from build123d import *

# Parameters (mm, degrees)
F1_DEPTH = 25.4
F2_R     = 7.2533857786
F2_R_2   = 5.5158705089
F2_R_3   = 6.7589997369
F2_R_4   = 6.3667286832
F2_R_5   = 6.9837940253
F2_R_6   = 6.9770855285
F3_DEPTH = 102.87
F4_R     = 5.2099395751
F5_DEPTH = 102.108
F9_START = 96.774
F9_DEPTH = 10.668


with BuildPart() as f1:
    # F0 (on Front) → F1 (new body)
    with BuildSketch(Plane.XZ):
        Polygon((-29.1519459024, 14.0827481248), (-26.7719905823, -18.2049516588), (2.3799553201, -32.2876997836), (29.1519459024, -14.0827481248), (26.7719905823, 18.2049516588), (-2.3799553201, 32.2876997836), align=None)
    extrude(amount=F1_DEPTH)

    # F2 (on Front) → F3 (join)
    with BuildSketch(Plane.XZ):
        with Locations((-28.9137475193, 13.9214349911)):
            Circle(F2_R)
        with Locations((-26.7719905823, -18.2049516588)):
            Circle(F2_R_2)
        with Locations((2.2947418038, -32.2793722153)):
            Circle(F2_R_3)
        with Locations((28.6077819765, -14.5333660766)):
            Circle(F2_R_4)
        with Locations((26.4660213143, 18.5109190643)):
            Circle(F2_R_5)
        with Locations((-2.9066735879, 32.5853340328)):
            Circle(F2_R_6)
    extrude(amount=F3_DEPTH)

    # F4 (on Front) → F5 (join)
    with BuildSketch(Plane.XZ):
        Circle(F4_R)
    extrude(amount=F5_DEPTH)

    # F6 (on Top) → F7 (revolve)
    with BuildSketch(Plane.XY):
        with BuildLine():
            Line((0, -67.7234342558), (0, -29.2267018693))
            ThreePointArc((0, -29.2267018693), (-19.2483661933, -48.4750680625), (0, -67.7234342558))
        make_face()
    revolve(axis=Axis((0, -48.4750680625, 0), (0, -1, 0)))

    # F8 (on Front) → F9 (join)
    with BuildSketch(Plane.XZ.offset(F9_START)):
        Polygon((-28.5810061773, 13.7057788732), (-26.1600557715, -17.8989879787), (2.4209504058, -31.6047668519), (28.5810061773, -13.7057788732), (26.1600557715, 17.8989879787), (-2.4209504058, 31.6047668519), align=None)
    extrude(amount=F9_DEPTH)


solid = f1.part
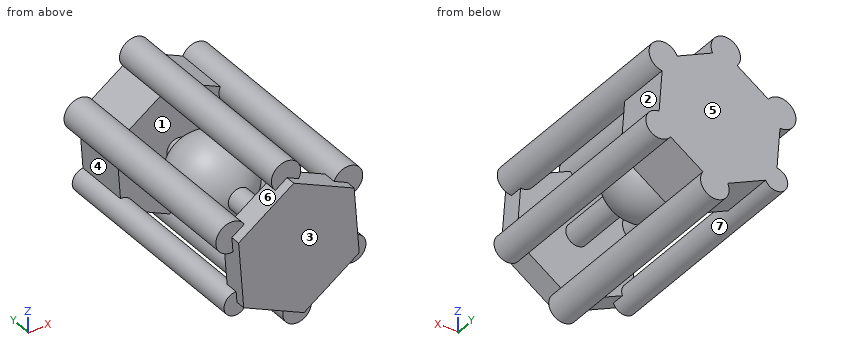
Source: CAD feature listing. Evaluate the final solid. Frame: model axes, mm. Face numbers are marked on the shaded views. A direction names the side the tool comes from. Round coordinates to 2 decimals unless told otherwise and drop trailing zeros. Loops run counter-clockwise (first coordinate to the right, second up) from the corner with the lowest first, then second, coordinate; pieces in that order, holes last. Notation, with made-up numbers: M 6,-39.5 L 61,-39.5 A23 cw 61,-8.5 Z; hole C 29,70 d11. An arc over 180 degrees is marked long. Return JSON: item names as keys, results as strings. Group by question number.
1. Mould query, pull axis Y, two halves, no side actions, for the marked faces 5, 6 and 7. Classes: released by +Y, released by -Y, zero draft, split by the parting line, or undercut.
2. Section query D-D on z = 0. Output: boundary loops of the cut face in (x, y).
3. Section query C-C on y = -16. Output: boundary loops of the cut face in (x, z), and give its area (3 significant figures).
4. Section query A-A on y = -27. Output: boundary loops of the cut face in (x, z), and give its area (3 significant figures).
5. Reachability of the marked faces 1, 2, 3 and 4 from +Z, -Z, +X, -X, +Y, -Y: full face, straight path, thin tool, end or side. Return the list, or none.
6. Pin query (flat end, axial travel): pin 1 (4 mm diameter, centred on x = 29.5, z = 17, fed in from -Y); pin 2 (3 mm diameter, centred on x = -2.5, y = -57.5, fed in from -Z); pin 3 (3 mm diameter, centred on x = -4, y = -11.5, fed in from -Z). Return the tip coordinate at first contact, or that it passes through.
7. Material intervals for line 1 along Z through (x, y) = (1, -44.5); line 2 along Y through (x, z) = (-15.5, 21); line 3 along Y through (x, z) = (-13.5, -9), sorted ascending. Write a range as from..to.
8. Section query B-B on x = -12.5. Output: boundary loops of the cut face in (y, z).
Checks:
{
 "1": {"face 5": "released by +Y", "face 6": "zero draft", "face 7": "undercut"},
 "2": {"outline": "M -28.11,-25.4 L -5.21,-25.4 L -5.21,-29.95 A19.25 ccw -5.21,-67 L -5.21,-96.77 L -27.53,-96.77 L -27.53,-107.44 L 27.53,-107.44 L 27.53,-96.77 L 5.21,-96.77 L 5.21,-67 A19.25 ccw 5.21,-29.95 L 5.21,-25.4 L 28.11,-25.4 L 28.11,0 L -28.11,0 Z"},
 "3": {"outline": "M -28.61,6.67 L -27.18,-12.7 A5.52 ccw long -21.81,-20.6 L -3.78,-29.31 A6.76 ccw long 7.91,-28.52 L 23.31,-18.06 A6.37 ccw long 28.72,-8.17 L 27.26,11.57 A6.98 ccw long 20.12,21.42 L 3.36,29.52 A6.98 ccw long -8.35,28.23 L -23.07,18.22 A7.25 ccw long Z", "area": "3,280 mm²"},
 "4": {"outline": "C -28.91,13.92 d14.51; C -26.77,-18.2 d11.03; C -2.91,32.59 d13.95; C 0,0 d10.42; C 2.29,-32.28 d13.52; C 26.47,18.51 d13.97; C 28.61,-14.53 d12.73", "area": "923 mm²"},
 "5": {"face 1": "none", "face 2": "+X, +Y, -Y", "face 3": "+Z, -Z, +X, -X, -Y", "face 4": "-X, +Y, -Y"},
 "6": {"pin 1": "stops at y = -102.87", "pin 2": "stops at z = -38.18", "pin 3": "stops at z = -37.04"},
 "7": {"line 1": "z = -38.91..-25.65, -18.81..18.81, 26.8..38.37", "line 2": "y = -107.44..-96.77, -25.4..0", "line 3": "y = -107.44..-96.77, -58.83..-38.12, -25.4..0"},
 "8": {"outline": "M -107.44,-24.45 L -96.77,-24.45 L -96.77,24.71 L -107.44,24.71 Z; C -48.48,0 d29.27; M -25.4,-25.1 L 0,-25.1 L 0,25.41 L -25.4,25.41 Z"}
}
